Geometry: final body of the model. Coordinates: model frame, mm. A direction names the side the tool comes from. Give positions to 0.01 mm unless a question says otherwise; leave off trailing zeros. Write each loop counter-clockwise with the first axis right and the second up, starting at its lowest first coordinate (ties: lowest second). Pieces come first, ordered by that corner, then holes. Notation, with made-up numbers: (8, 77) -> (20, 77) arc R20 ccw to (20, 92) -> close; hole circle Ø9 at (76.5, 80). An arc over 180 degrees is marked (long way). Answer in a Markdown table with one row per item. Add a question column.
Item 1: Material intervals for probe 1 along X at (y, z) = (-98, 804.5); probe 2 along Z at (x, y) = (203.5, -71); probe 3 along X at (y, z) = (58, 57), sorted ascending. Write a range as from..to.
Item 2: Section query A-A on x = 338.5. Output: boundary loops of the cut face in (y, z).
Item 3: Section query C-C on y = -88.5. Output: boundary loops of the cut face in (x, z), plus the area to 3 significant figures.
Item 4: Section query B-B on z = 1278. Output: boundary loops of the cut face in (x, y).
Item 5: Draft query along X for faces 5 (the flat face through (495.3, 442, 1007)), 6 (the flat face through (-7, 430, 0)), 7 (the flat face through (-525, 1041.4, 100)), 8 (the flat face through (406.4, -69, 1002)). Return one class per face: +X half, -X half, draft (parallel to the pull), parting line (faces both ways), or undercut.
Item 6: First-contact query: P1, Ø12, axis at y = 120.5, z = 391, coming from the -X side; P2, Ø4, axis at x = 31.5, y = -7, coming from the +Z side. Flat tips, straight axial feed; report the tip coordinate or a pass-through.
Item 7: Access query for faces 1 (the flat face through (-374.65, 526, 100)), 2 (the flat face through (389, -139.7, 1322)), 3 (the flat face through (374.65, -69, 1004)), 4 (the flat face through (389, 0, 1322)). Directions: +Z, -Z, +X, -X, +Y, -Y. A direction counts if a zero-diameter tool reaches every point of the face in a straight line with its end or side. Return the directions, or none.
Item 8: Section query D-D on y = 62.5. Output: boundary loops of the cut face in (x, z), plus the area to 3 significant figures.
```python
from build123d import *

# Parameters (mm, degrees)
F1_DEPTH = 139.7
F2_W     = 939.8
F2_H     = 1206.5
F3_DEPTH = 152.4
F4_W     = 939.8
F4_H     = 2286
F5_DEPTH = 25.4
F6_W     = 1231.9
F6_H     = 2286
F7_DEPTH = 25.4
F8_W     = 203.2
F8_H     = 1016
F9_DEPTH = 203.2


with BuildPart() as f1:
    # F0 (on Front) → F1 (new body)
    with BuildSketch(Plane.XZ):
        Polygon((-374.65, 0), (-374.65, 1981.2), (374.65, 1981.2), (374.65, 0), (406.4, 0), (406.4, 2032), (-406.4, 2032), (-406.4, 0), align=None)
    extrude(amount=F1_DEPTH)

    # F2 (on face) → F3 (join)
    with BuildSketch(Plane(origin=(0, 0, 0), x_dir=(1, 0, 0), z_dir=(0, 0, -1))):
        with Locations((0, -438.15)):
            Rectangle(F2_W, F2_H)
    extrude(amount=F3_DEPTH)

    # F4 (on face) → F5 (join)
    with BuildSketch(Plane(origin=(0, 1041.4, 0), x_dir=(-1, 0, 0), z_dir=(0, 1, 0))):
        with Locations((0, 990.6)):
            Rectangle(F4_W, F4_H)
    extrude(amount=F5_DEPTH)

    # F6 (on face) → F7 (join)
    with BuildSketch(Plane.YZ.offset(469.9)):
        with Locations((450.85, 990.6)):
            Rectangle(F6_W, F6_H)
    extrude(amount=F7_DEPTH)

    # F8 (on face) → F9 (join)
    with BuildSketch(Plane.XY):
        with Locations((-476.25, 533.4)):
            Rectangle(F8_W, F8_H)
    extrude(amount=F9_DEPTH)


solid = f1.part
```
Findings below:
| question | item | result |
|---|---|---|
| 1 | probe 1 | x = -406.4..-374.65, 374.65..406.4, 469.9..495.3 |
| 1 | probe 2 | z = -152.4..0, 1981.2..2032 |
| 1 | probe 3 | x = -577.85..-374.65, 469.9..495.3 |
| 2 | outline | (-165.1, -152.4) -> (1066.8, -152.4) -> (1066.8, 2133.6) -> (1041.4, 2133.6) -> (1041.4, 0) -> (-165.1, 0) -> close; (-139.7, 1981.2) -> (0, 1981.2) -> (0, 2032) -> (-139.7, 2032) -> close |
| 3 | outline | (-469.9, -152.4) -> (495.3, -152.4) -> (495.3, 2133.6) -> (469.9, 2133.6) -> (469.9, 0) -> (406.4, 0) -> (406.4, 2032) -> (-406.4, 2032) -> (-406.4, 0) -> (-469.9, 0) -> close; hole (-374.65, 0) -> (374.65, 0) -> (374.65, 1981.2) -> (-374.65, 1981.2) -> close |
| 3 | area | 368,000 mm^2 |
| 4 | outline | (-469.9, 1041.4) -> (469.9, 1041.4) -> (469.9, -165.1) -> (495.3, -165.1) -> (495.3, 1066.8) -> (-469.9, 1066.8) -> close; (-406.4, -139.7) -> (-374.65, -139.7) -> (-374.65, 0) -> (-406.4, 0) -> close; (374.65, -139.7) -> (406.4, -139.7) -> (406.4, 0) -> (374.65, 0) -> close |
| 5 | face 5 | +X half |
| 5 | face 6 | undercut |
| 5 | face 7 | draft |
| 5 | face 8 | undercut |
| 6 | P1 | stops at x = 469.9 |
| 6 | P2 | stops at z = 2032 |
| 7 | face 1 | +Z, -Y |
| 7 | face 2 | +Z, -X, -Y |
| 7 | face 3 | -Y |
| 7 | face 4 | +Z, -X |
| 8 | outline | (-577.85, 0) -> (-469.9, 0) -> (-469.9, -152.4) -> (495.3, -152.4) -> (495.3, 2133.6) -> (469.9, 2133.6) -> (469.9, 0) -> (-374.65, 0) -> (-374.65, 203.2) -> (-577.85, 203.2) -> close |
| 8 | area | 243,000 mm^2 |
